The model under review builds one solid part; all positions refer to its coordinate system, in mm. Coordinates: 2 decimals unless noted, no trailing zeros. Put each result on its own line as item: value.
from build123d import *

# Parameters (mm, degrees)
BOSS_EXTRUDE1_DEPTH = 5
FILLET1_R           = 10
SHELL1_T            = -1
SKETCH4_R           = 1
CUT_EXTRUDE1_DEPTH  = 15.976807967


with BuildPart() as part:
    # Sketch1 → Boss-Extrude1 (new body)
    with BuildSketch(Plane.XY):
        with BuildLine():
            ThreePointArc((-0.15625, 9.998779222), (-10, 0), (-0.15625, -9.998779222))
            ThreePointArc((-0.15625, -9.998779222), (-2.5, 0), (-0.15625, 9.998779222))
        make_face()
    extrude(amount=BOSS_EXTRUDE1_DEPTH)

    # Fillet1
    # the kernel refuses this fillet: 10 mm, written as the material it takes off along each edge
    with BuildSketch(Plane(origin=(0, 0, 5), x_dir=(0.9999950652018581, 0.003141587485880102, 0), z_dir=(0.003141587485880102, -0.9999950652018581, 0))) as fillet1_piece_1:
        with BuildLine():
            CenterArc((1.339745962, -10), FILLET1_R, 30, 60)
            Line((1.339745962, 0), (1.339745962, 0.2))
            Line((1.339745962, 0.2), (10, 0.2))
            Line((10, 0.2), (10.2, 0))
            ThreePointArc((10.2, 0), (10.2, -2.5), (10.173205081, -4.9))
            Line((10.173205081, -4.9), (10, -5))
        make_face()
    revolve(axis=Axis((0, 0, 5), (0, 0, 1)), revolution_arc=359.64, mode=Mode.SUBTRACT)

    # Shell1
    shell1_openings = [part.faces().sort_by_distance(p)[0] for p in [
        (-5.162614347, 0, 0),
    ]]
    offset(amount=SHELL1_T, openings=shell1_openings, kind=Kind.INTERSECTION)

    # Sketch4 → Cut-Extrude1 (cut, through all)
    with BuildSketch(Plane(origin=(0, 0, 0), x_dir=(0, 0, -1), z_dir=(1, 0, 0))):
        with Locations(Location((-2.466231233, 0, 0), (0, 0, 324.775001353))):
            Circle(SKETCH4_R)
    extrude(amount=-CUT_EXTRUDE1_DEPTH, mode=Mode.SUBTRACT)


solid = part.part
1. The part is to be moulded in two halves that separate along Z. For faces 1 (the flat face through (-3, 0, 0)), 2 (the cylindrical face through (-6.65, -0.67, 3.21)), say which applies: +Z half, -Z half, draft (parallel to the pull), parting line (faces both ways), or undercut.
Determined:
face 1: -Z half
face 2: undercut
2. To check wall thickness, follow probe 1 along X at (y, z) = (5.5, 1.4); probe 2 along Y at (x, z) = (-5.5, 1.35); probe 3 along Y at (x, z) = (-5.75, 1.7). State the ranges of each line that lie inside material, in increasing order.
Determined:
probe 1: x = -7.15 to -5.34, -2.85 to -1.82
probe 2: y = -7.21 to -5.41, 5.41 to 7.21
probe 3: y = -6.61 to -4.58, 4.58 to 6.61
3. For pin 1 Ø2.5 at (y, z) = (0, 2.47) entering from -X; pin 2 Ø1.6 at (y, z) = (0, 2.47) entering from -X; pin 3 Ø3 at (x, y) = (-2.5, -3) entering from +Z, all flat-tipped, find the tip position at first contact; note any pin that passes through.
Determined:
pin 1: stops at x = -9.17
pin 2: passes through
pin 3: stops at z = 4.88
4. Consider section A-A on y = 0. Give the number of separate pieces and of enclosed holes in the cut face, plus the area to 3 significant figures.
Determined:
separate pieces: 3
enclosed holes: 0
area: 6.96 mm^2
